Here's how the part is built. I have some questions about the finished solid (model axes, mm). A direction names the side the tool comes from. Coordinates: 2 decimals unless noted, no trailing zeros. Write each loop counter-clockwise with the first axis right and the second up, starting at its lowest first coordinate (ties: lowest second). Pieces come first, ordered by that corner, then holes. Notation, with made-up numbers: (82.5, 67) -> (126.5, 67) arc R21 ccw to (126.5, 100) -> close; hole circle Ø9 at (-26.5, 70.25). An arc over 180 degrees is marked (long way). Put each result on its own line as item: value.
```python
from build123d import *

# Parameters (mm, degrees)
F1_DEPTH = 1.8
F2_R     = 0.25
F3_R     = 0.25


with BuildPart() as f1:
    # F0 (on Front) → F1 (new body)
    with BuildSketch(Plane.XZ):
        Polygon((8, 3.50676), (-4.5, 1.75), (-8.5, 2), (-8.5, 3), (-9.5, 3), (-9.5, 1.5), (-5, 0), (-9.5, -1.5), (-9.5, -3), (-8.5, -3), (-8.5, -2), (-4.5, -1.75), (8, -3.50676), (8, -1.68649), (-4, 0), (8, 1.68649), align=None)
    extrude(amount=F1_DEPTH)

    # F2
    f2_edges = [f1.edges().sort_by_distance(p)[0] for p in [
        (-4, -0.9, 0),
        (-5, -0.9, 0),
    ]]
    fillet(f2_edges, radius=F2_R)

    # F3
    f3_edges = [f1.edges().sort_by_distance(p)[0] for p in [
        (-8.5, -0.9, 2),
        (-8.5, -0.9, -2),
    ]]
    fillet(f3_edges, radius=F3_R)


solid = f1.part
```
Item 1: Imagine slicing it at A-A on x = -1. Write out the boundary of the cut face in (y, z), then the cut area to 3 significant figures.
Output:
outline: (-1.8, -2.24) -> (0, -2.24) -> (0, -0.42) -> (-1.8, -0.42) -> close; (-1.8, 0.42) -> (0, 0.42) -> (0, 2.24) -> (-1.8, 2.24) -> close
area: 6.55 mm²
Item 2: Imagine slicing it at B-B on z = -2.5. Write out the boundary of the cut face in (x, y).
Output:
outline: (-9.5, -1.8) -> (-8.5, -1.8) -> (-8.5, 0) -> (-9.5, 0) -> close; (0.84, -1.8) -> (8, -1.8) -> (8, 0) -> (0.84, 0) -> close
Item 3: If we mould it in two halves opening along X, with no side actions, what happens to faces 6 (the flat face through (-9.5, -1, 2)), 7 (the flat face through (-9, -1, 3)), 8 (the flat face through (1.663, -0.887, -2.616))? For each: released by +X, released by -X, zero draft, split by the parting line, or undercut.
Output:
face 6: released by -X
face 7: zero draft
face 8: undercut
Item 4: Imagine slicing it at C-C on y = -0.45. Write out the boundary of the cut face in (x, z).
Output:
outline: (-9.5, -3) -> (-8.5, -3) -> (-8.5, -2.23) arc R0.25 cw to (-8.27, -1.99) -> (-4.5, -1.75) -> (8, -3.51) -> (8, -1.69) -> (-2.24, -0.25) arc R0.25 cw to (-2.24, 0.25) -> (8, 1.69) -> (8, 3.51) -> (-4.5, 1.75) -> (-8.27, 1.99) arc R0.25 cw to (-8.5, 2.23) -> (-8.5, 3) -> (-9.5, 3) -> (-9.5, 1.5) -> (-5.71, 0.24) arc R0.25 cw to (-5.71, -0.24) -> (-9.5, -1.5) -> close
Item 5: Imagine slicing it at D-D on z = 0. Write out the boundary of the cut face in (x, y), then the cut area to 3 significant figures.
Output:
outline: (-5.54, -1.8) -> (-2.45, -1.8) -> (-2.45, 0) -> (-5.54, 0) -> close
area: 5.56 mm²
Item 6: Please list where these lines run through material, in increasing order: line 1 along Z through (x, y) = (2, -0.4); line 2 along Z through (x, y) = (3, -0.2); line 3 along Z through (x, y) = (-2.5, -1.2). Write a range as from..to.
Output:
line 1: z = -2.66..-0.84, 0.84..2.66
line 2: z = -2.8..-0.98, 0.98..2.8
line 3: z = -2.03..2.03
Item 7: Which directions (+Z, -Z, +X, -X, +Y, -Y) give clear straight access to the entire face, cutting with the end or side of a thin tool? Please do faces 1 (the flat face through (-9, -1, -3)), 2 (the flat face through (-6.41, -0.89, -1.87)), 3 (the flat face through (-8, -1, -1)), 4 (the flat face through (2.952, -0.887, -0.977)), 5 (the flat face through (1.84, -0.89, 2.64)).
Output:
face 1: -Z, -X, +Y, -Y
face 2: -Z, +Y, -Y
face 3: -X, +Y, -Y
face 4: +X, +Y, -Y
face 5: +Z, +Y, -Y
Item 8: For P1, Ø0.8, axis at x = -9, y = -1, coming from the +Z side; P2, Ø2, axis at x = -1, z = 0, coming from the -Y side; P3, Ø0.8, axis at x = -9, y = -1, coming from the -Z side, each with a flat end and sliding along its axis, tell me the tip position at first contact or that it passes through.
Output:
P1: stops at z = 3
P2: stops at y = -1.8
P3: stops at z = -3
